```python
from build123d import *

# Parameters (mm, degrees)
SKETCH1_R           = 1.6
BOSS_EXTRUDE1_DEPTH = 1.5
SKETCH2_W           = 21.020817279
SKETCH2_H           = 13.668708773
SKETCH2_W_2         = 16.538575955
SKETCH2_H_2         = 13.76502595
SKETCH2_H_3         = 12.635061133
BOSS_EXTRUDE2_DEPTH = 10
SKETCH3_W           = 17.580136513
SKETCH3_H           = 16.463937369
BOSS_EXTRUDE3_DEPTH = 5
SKETCH4_W           = 7
SKETCH4_H           = 10.668708773
CUT_EXTRUDE1_DEPTH  = 15
SKETCH5_W           = 3.25
SKETCH5_H           = 10.635061133
SKETCH5_H_2         = 11.76502595
CUT_EXTRUDE2_DEPTH  = 15


with BuildPart() as part:
    # Sketch1 → Boss-Extrude1 (new body)
    with BuildSketch(Plane.XY):
        with BuildLine():
            Line((7.342063859, 25.576361327), (86.342063859, 25.576361327))
            ThreePointArc((86.342063859, 25.576361327), (88.463384202, 24.697681671), (89.342063859, 22.576361327))
            Line((89.342063859, 22.576361327), (89.342063859, -26.423638673))
            ThreePointArc((89.342063859, -26.423638673), (88.463384202, -28.544959016), (86.342063859, -29.423638673))
            Line((86.342063859, -29.423638673), (7.342063859, -29.423638673))
            ThreePointArc((7.342063859, -29.423638673), (5.220743515, -28.544959016), (4.342063859, -26.423638673))
            Line((4.342063859, -26.423638673), (4.342063859, 22.576361327))
            ThreePointArc((4.342063859, 22.576361327), (5.220743515, 24.697681671), (7.342063859, 25.576361327))
        make_face()
        with Locations((7.342063859, 22.576361327)):
            Circle(SKETCH1_R, mode=Mode.SUBTRACT)
        with Locations((7.342063859, -26.423638673)):
            Circle(SKETCH1_R, mode=Mode.SUBTRACT)
        with Locations((65.342063859, -26.423638673)):
            Circle(SKETCH1_R, mode=Mode.SUBTRACT)
        with Locations((65.342063859, 22.576361327)):
            Circle(SKETCH1_R, mode=Mode.SUBTRACT)
    extrude(amount=BOSS_EXTRUDE1_DEPTH)

    # Sketch2 → Boss-Extrude2 (add)
    with BuildSketch(Plane.XY.offset(1.5)):
        with Locations((82.249107191, 13.642831506)):
            Rectangle(SKETCH2_W, SKETCH2_H)
        with Locations((82.18632648, -2.437513953)):
            Rectangle(SKETCH2_W_2, SKETCH2_H_2)
        with Locations((82.18632648, -17.281142683)):
            Rectangle(SKETCH2_W_2, SKETCH2_H_3)
    extrude(amount=BOSS_EXTRUDE2_DEPTH)

    # Sketch3 → Boss-Extrude3 (add)
    with BuildSketch(Plane.XY.offset(1.5)):
        with Locations((38.810601532, -0.796926727)):
            Rectangle(SKETCH3_W, SKETCH3_H)
    extrude(amount=BOSS_EXTRUDE3_DEPTH)

    # Sketch4 → Cut-Extrude1 (cut)
    with BuildSketch(Plane(origin=(92.75951583, 0, 0), x_dir=(0, 0, -1), z_dir=(1, 0, 0))):
        with Locations((-6.5, 13.642831506)):
            Rectangle(SKETCH4_W, SKETCH4_H)
    extrude(amount=-CUT_EXTRUDE1_DEPTH, mode=Mode.SUBTRACT)

    # Sketch5 → Cut-Extrude2 (cut)
    with BuildSketch(Plane(origin=(90.455614457, 0, 0), x_dir=(0, 0, -1), z_dir=(1, 0, 0))):
        with Locations((-4.125, -17.281142683)):
            Rectangle(SKETCH5_W, SKETCH5_H)
        with Locations((-8.875, -17.281142683)):
            Rectangle(SKETCH5_W, SKETCH5_H)
        with Locations((-4.125, -2.437513953)):
            Rectangle(SKETCH5_W, SKETCH5_H_2)
        with Locations((-8.875, -2.437513953)):
            Rectangle(SKETCH5_W, SKETCH5_H_2)
    extrude(amount=-CUT_EXTRUDE2_DEPTH, mode=Mode.SUBTRACT)


solid = part.part
```
Check sheet for the modelled part. Datum: model origin and axes. Units: mm. A direction names the side the tool comes from. Round coordinates to 2 decimals unless told otherwise and drop trailing zeros. Loops run counter-clockwise (first coordinate to the right, second up) from the corner with the lowest first, then second, coordinate; pieces in that order, holes last. Notation, with made-up numbers: (41, 69) - (70, 69) arc R22 ccw to (70, 81) - close; hole circle Ø4 at (17, -7.5). An arc over 180 degrees is marked (long way). Answer as a JSON object with one key per item and string values. Group by question number.
Q1. Sectioned sample at D-D, the plane x = 31. Enter the section's corners in (y, z), plus the area to 3 significant figures.
Q2. Mould release check, pull along Z, two halves, no side actions. Record for faces 6 (the face through (85, 18.977, 7)), 7 (the face through (82, -23.599, 6)), 8 (the face through (82, -17, 11.5)): released by +Z, released by -Z, zero draft, split by the parting line, or undercut.
Q3. Sectioned sample at A-A, the plane z = 4. Enter the section's corners in (x, y) (3 decimals), plus the area to 3 significant figures.
Q4. Scan lines: line 1 along Z through (x, y) = (83.5, -4); line 2 along X through (y, z) = (-3.5, 2); line 3 along X through (y, z) = (7, 4). Record each from-to range of solid material in increasing order. Write a range as [from, to].
Q5. Sectioned sample at B-B, the plane z = 8.25. Enter the section's corners in (x, y) (3 decimals), plus the area to 3 significant figures.
Q6. Set-up check for faces 1 (the face through (82, -10.964, 6)), 2 (the face through (75.456, -2, 9)), 3 (the face through (47.601, -1, 4)), 4 (the face through (91, 14, 1.5)), 5 (the face through (5.244, -28.568, 0.74)): record each of +Z, -Z, +X, -X, +Y, -Y from which the full face is reachable in a straight line by a thin tool's end or side.
Q7. Sectioned sample at C-C, the plane y = -6. Enter the section's corners in (x, z), plus the area to 3 significant figures.
Q8. Gauge pin test, flat ends, axial feed: P1, Ø3.5, axis at y = -16, z = 9.5, coming from the +X side; P2, Ø5, axis at y = 1, z = 7.5, coming from the -X side; P3, Ø5, axis at x = 78.5, z = 9, coming from the -Y side; P4, Ø3, axis at x = 18, z = 4.5, coming from the +Y side. Record the tip position at first contact, or that the pin passes through.
Solution:
{
 "1": {"outline": "(-29.42, 0) - (25.58, 0) - (25.58, 1.5) - (7.44, 1.5) - (7.44, 6.5) - (-9.03, 6.5) - (-9.03, 1.5) - (-29.42, 1.5) - close", "area": "165 mm²"},
 "2": {"face 6": "undercut", "face 7": "zero draft", "face 8": "released by +Z"},
 "3": {"outline": "(30.021, -9.029) - (47.601, -9.029) - (47.601, 7.435) - (30.021, 7.435) - close; (71.739, 6.808) - (92.76, 6.808) - (92.76, 8.308) - (77.76, 8.308) - (77.76, 18.977) - (92.76, 18.977) - (92.76, 20.477) - (71.739, 20.477) - close; (73.917, -23.599) - (90.456, -23.599) - (90.456, -22.599) - (75.456, -22.599) - (75.456, -11.964) - (90.456, -11.964) - (90.456, -10.964) - (73.917, -10.964) - close; (73.917, -9.32) - (90.456, -9.32) - (90.456, -8.32) - (75.456, -8.32) - (75.456, 3.445) - (90.456, 3.445) - (90.456, 4.445) - (73.917, 4.445) - close", "area": "517 mm²"},
 "4": {"line 1": "z = [0, 2.5], [5.75, 7.25], [10.5, 11.5]", "line 2": "x = [30.02, 47.6], [73.92, 90.46]", "line 3": "x = [30.02, 47.6], [71.74, 92.76]"},
 "5": {"outline": "(71.739, 6.808) - (92.76, 6.808) - (92.76, 8.308) - (77.76, 8.308) - (77.76, 18.977) - (92.76, 18.977) - (92.76, 20.477) - (71.739, 20.477) - close; (73.917, -23.599) - (90.456, -23.599) - (90.456, -22.599) - (75.456, -22.599) - (75.456, -11.964) - (90.456, -11.964) - (90.456, -10.964) - (73.917, -10.964) - close; (73.917, -9.32) - (90.456, -9.32) - (90.456, -8.32) - (75.456, -8.32) - (75.456, 3.445) - (90.456, 3.445) - (90.456, 4.445) - (73.917, 4.445) - close", "area": "228 mm²"},
 "6": {"face 1": "+Z, +X, -X", "face 2": "+X", "face 3": "+Z, +Y, -Y", "face 4": "-Z, +X, +Y, -Y", "face 5": "+Z, -Z, -X, -Y"},
 "7": {"outline": "(4.34, 0) - (89.34, 0) - (89.34, 1.5) - (90.46, 1.5) - (90.46, 2.5) - (75.46, 2.5) - (75.46, 5.75) - (90.46, 5.75) - (90.46, 7.25) - (75.46, 7.25) - (75.46, 10.5) - (90.46, 10.5) - (90.46, 11.5) - (73.92, 11.5) - (73.92, 1.5) - (47.6, 1.5) - (47.6, 6.5) - (30.02, 6.5) - (30.02, 1.5) - (4.34, 1.5) - close", "area": "283 mm²"},
 "8": {"P1": "stops at x = 90.46", "P2": "stops at x = 30.02", "P3": "stops at y = -23.6", "P4": "passes through"}
}
